Geometry check sheet. Reference: the model listing, model coordinates, mm. A direction names the side the tool comes from. Round coordinates to 2 decimals unless told otherwise and drop trailing zeros. Order: outer loops, then holes, each group sorted by start corner. A loop starts at its lowest first (then second) coordinate and runs counter-clockwise, first axis right, second up.
```python
from build123d import *

# Parameters (mm, degrees)
FILLET1_R = 4.7625


with BuildPart() as part:
    # Sketch1 → Revolve1 (revolve)
    with BuildSketch(Plane.XY, mode=Mode.PRIVATE) as revolve1_sk:
        Polygon((257.175, 0), (257.175, 15.113), (250.063, 15.113), (245.237, 31.877), (29.718, 31.877), (29.718, 34.417), (21.336, 34.798), (12.954, 30.988), (7.9502, 15.113), (0, 15.113), (0, 0), align=None)
    revolve(revolve1_sk.sketch.rotate(Axis((0, 0, 0), (1, 0, 0)), 90), axis=Axis((0, 0, 0), (1, 0, 0)))

    # Fillet1
    fillet1_edges = [part.edges().sort_by_distance(p)[0] for p in [
        (12.954, 0, -30.988),
        (245.237, 0, -31.877),
    ]]
    fillet(fillet1_edges, radius=FILLET1_R)


solid = part.part
```
(1) Depth check by flat-ended pin: P1, Ø1.5, axis at x = 207.5, y = -14.5, coming from the -Z side; P2, Ø4, axis at y = -20, z = 15, coming from the +X side; P3, Ø5, axis at x = 134, z = -2, coming from the +Y side. Enter the tip coordinate at first touch or a pass-through.
Returned:
P1: stops at z = -28.76
P2: stops at x = 247.79
P3: stops at y = 31.88
(2) Material ranges on line 1 (Z direction, x = 77, y = -1); line 2 (Z direction, x = 170.5, y = 21.5); line 3 (X direction, y = 9.5, z = -25.5), recorded low to high.
Returned:
line 1: z = -31.86 to 31.86
line 2: z = -23.53 to 23.53
line 3: x = 11.76 to 246.58
(3) Set-up check for faces 1 (the cylindrical face through (3.919, -4.54, 14.415)), 2 (the flat face through (0, 0, 0)), 3 (the cylindrical face through (134.202, -9.575, 30.405)): record each of +Z, -Z, +X, -X, +Y, -Y from which the full face is reachable in a straight line by a thin tool's end or side.
Returned:
face 1: -X
face 2: +Z, -Z, -X, +Y, -Y
face 3: +X
(4) Sectioned sample at A-A, the plane x = 155.5. Record the cut outline in (y, z).
Returned:
outline: circle Ø63.75 at (0, 0)
